Geometry: final body of the model. Coordinates: model frame, mm. Face numbers are marked on the shaded views. A direction names the side the tool comes from. Round coordinates to 2 decimals unless told otherwise and drop trailing zeros. Order: outer loops, then holes, each group sorted by start corner. A loop starts at its lowest first (then second) coordinate and runs counter-clockwise, first axis right, second up. Notation, with made-up numbers: (-8.75, 79) -> (23.25, 79) arc R30 ccw to (23.25, 117) -> close; hole circle Ø8 at (83, 64). An arc over 180 degrees is marked (long way). Put each result on its own line as item: value.
```python
from build123d import *

# Parameters (mm, degrees)
F1_DEPTH = 10
F2_DEPTH = 50
F3_DEPTH = 10
F4_START = 50
F4_DEPTH = 10


# Not quite as in the source:
# - a feature names something its author has since deleted; it is built from what else it names


with BuildPart() as f1:
    # F0 (on Top) → F1 (new body)
    with BuildSketch(Plane.XY):
        with BuildLine():
            Line((0, 11.5), (0, 14))
            ThreePointArc((0, 14), (-14, 0), (0, -14))
            Line((0, -14), (0, -11.5))
            ThreePointArc((0, -11.5), (-2.4269719101, -11.2409878279), (-4.7446194261, -10.4756186692))
            ThreePointArc((-4.7446194261, -10.4756186692), (-8.9623106012, -8.9623106012), (-10.4756186692, -4.7446194261))
            ThreePointArc((-10.4756186692, -4.7446194261), (-11.5, 0), (-10.4756186692, 4.7446194261))
            ThreePointArc((-10.4756186692, 4.7446194261), (-8.9623106012, 8.9623106012), (-4.7446194261, 10.4756186692))
            ThreePointArc((-4.7446194261, 10.4756186692), (-2.4269719101, 11.2409878279), (0, 11.5))
        make_face()
        with BuildLine():
            ThreePointArc((-4.7446194261, -10.4756186692), (-2.4269719101, -11.2409878279), (0, -11.5))
            Line((0, -11.5), (0, -9))
            Line((0, -9), (0, -5.25))
            ThreePointArc((0, -5.25), (-1.3631151282, -8.7791112186), (-4.7446194261, -10.4756186692))
        make_face()
        with BuildLine():
            Line((-5.25, -5.25), (0, -5.25))
            ThreePointArc((0, -5.25), (-0.001489151, -5.124964534), (-0.0059557591, -5))
            Line((-0.0059557591, -5), (-3, -5))
            Line((-3, -5), (-3, -0.5065835097))
            ThreePointArc((-3, -0.5065835097), (-4.0968383837, -0.1282114172), (-5.2499999999, 0))
            Line((-5.25, 0), (-5.25, -5.25))
        make_face()
        with BuildLine():
            ThreePointArc((-10.4756186692, -4.7446194261), (-8.1317279836, -8.1317279836), (-4.7446194261, -10.4756186692))
            ThreePointArc((-4.7446194261, -10.4756186692), (-1.3631151282, -8.7791112186), (0, -5.25))
            Line((0, -5.25), (-5.25, -5.25))
            Line((-5.25, -5.25), (-5.25, 0))
            ThreePointArc((-5.2499999999, 0), (-8.7791112186, -1.3631151282), (-10.4756186692, -4.7446194261))
        make_face()
        with BuildLine():
            ThreePointArc((-5.2499999999, 0), (-8.7791112186, 1.3631151282), (-10.4756186692, 4.7446194261))
            ThreePointArc((-10.4756186692, 4.7446194261), (-11.5, 0), (-10.4756186692, -4.7446194261))
            ThreePointArc((-10.4756186692, -4.7446194261), (-8.7791112186, -1.3631151282), (-5.2499999999, 0))
        make_face()
        with BuildLine():
            ThreePointArc((-3, 0.5065835097), (-4.0968383837, 0.1282114172), (-5.2499999999, 0))
            ThreePointArc((-5.2499999999, 0), (-4.0968383837, -0.1282114172), (-3, -0.5065835097))
            Line((-3, -0.5065835097), (-3, 0.5065835097))
        make_face()
        with BuildLine():
            ThreePointArc((0, 5.25), (-1.3631151282, 8.7791112186), (-4.7446194261, 10.4756186692))
            ThreePointArc((-4.7446194261, 10.4756186692), (-8.1317279836, 8.1317279836), (-10.4756186692, 4.7446194261))
            ThreePointArc((-10.4756186692, 4.7446194261), (-8.7791112186, 1.3631151282), (-5.2499999999, 0))
            Line((-5.25, 0), (-5.25, 5.25))
            Line((-5.25, 5.25), (0, 5.25))
        make_face()
        with BuildLine():
            Line((0, 9), (0, 11.5))
            ThreePointArc((0, 11.5), (-2.4269719101, 11.2409878279), (-4.7446194261, 10.4756186692))
            ThreePointArc((-4.7446194261, 10.4756186692), (-1.3631151282, 8.7791112186), (0, 5.25))
            Line((0, 5.25), (0, 6))
            Line((0, 6), (0, 9))
        make_face()
        with BuildLine():
            ThreePointArc((-10.4756186692, 4.7446194261), (-8.1317279836, 8.1317279836), (-4.7446194261, 10.4756186692))
            ThreePointArc((-4.7446194261, 10.4756186692), (-8.9623106012, 8.9623106012), (-10.4756186692, 4.7446194261))
        make_face()
        with BuildLine():
            ThreePointArc((-10.4756186692, -4.7446194261), (-8.9623106012, -8.9623106012), (-4.7446194261, -10.4756186692))
            ThreePointArc((-4.7446194261, -10.4756186692), (-8.1317279836, -8.1317279836), (-10.4756186692, -4.7446194261))
        make_face()
        with BuildLine():
            ThreePointArc((-0.0059557591, 5), (-0.001489151, 5.124964534), (0, 5.25))
            Line((0, 5.25), (-5.25, 5.25))
            Line((-5.25, 5.25), (-5.25, 0))
            ThreePointArc((-5.2499999999, 0), (-4.0968383837, 0.1282114172), (-3, 0.5065835097))
            Line((-3, 0.5065835097), (-3, 5))
            Line((-3, 5), (-0.0059557591, 5))
        make_face()
    extrude(amount=-F1_DEPTH)

    # F0 (on Top) → F2 (join)
    with BuildSketch(Plane.XY):
        with BuildLine():
            Line((0, 11.5), (0, 14))
            ThreePointArc((0, 14), (-14, 0), (0, -14))
            Line((0, -14), (0, -11.5))
            ThreePointArc((0, -11.5), (-2.4269719101, -11.2409878279), (-4.7446194261, -10.4756186692))
            ThreePointArc((-4.7446194261, -10.4756186692), (-8.9623106012, -8.9623106012), (-10.4756186692, -4.7446194261))
            ThreePointArc((-10.4756186692, -4.7446194261), (-11.5, 0), (-10.4756186692, 4.7446194261))
            ThreePointArc((-10.4756186692, 4.7446194261), (-8.9623106012, 8.9623106012), (-4.7446194261, 10.4756186692))
            ThreePointArc((-4.7446194261, 10.4756186692), (-2.4269719101, 11.2409878279), (0, 11.5))
        make_face()
    extrude(amount=F2_DEPTH)

    # F3 (add): a face of the model
    f3_faces = [f1.faces().sort_by_distance(p)[0] for p in [
        (-2.4930382043, 11.5469865939, 50),
    ]]
    extrude(f3_faces, amount=F3_DEPTH)

    # F0 (on Top) → F4 (join)
    with BuildSketch(Plane.XY.offset(F4_START)):
        with BuildLine():
            Line((0, 9), (0, 11.5))
            ThreePointArc((0, 11.5), (-2.4269719101, 11.2409878279), (-4.7446194261, 10.4756186692))
            ThreePointArc((-4.7446194261, 10.4756186692), (-1.3631151282, 8.7791112186), (0, 5.25))
            Line((0, 5.25), (0, 6))
            Line((0, 6), (0, 9))
        make_face()
        with BuildLine():
            ThreePointArc((-4.7446194261, -10.4756186692), (-2.4269719101, -11.2409878279), (0, -11.5))
            Line((0, -11.5), (0, -9))
            Line((0, -9), (0, -5.25))
            ThreePointArc((0, -5.25), (-1.3631151282, -8.7791112186), (-4.7446194261, -10.4756186692))
        make_face()
        with BuildLine():
            ThreePointArc((0, 5.25), (-1.3631151282, 8.7791112186), (-4.7446194261, 10.4756186692))
            ThreePointArc((-4.7446194261, 10.4756186692), (-8.1317279836, 8.1317279836), (-10.4756186692, 4.7446194261))
            ThreePointArc((-10.4756186692, 4.7446194261), (-8.7791112186, 1.3631151282), (-5.2499999999, 0))
            Line((-5.25, 0), (-5.25, 5.25))
            Line((-5.25, 5.25), (0, 5.25))
        make_face()
        with BuildLine():
            ThreePointArc((-10.4756186692, 4.7446194261), (-8.1317279836, 8.1317279836), (-4.7446194261, 10.4756186692))
            ThreePointArc((-4.7446194261, 10.4756186692), (-8.9623106012, 8.9623106012), (-10.4756186692, 4.7446194261))
        make_face()
        with BuildLine():
            ThreePointArc((-10.4756186692, -4.7446194261), (-8.9623106012, -8.9623106012), (-4.7446194261, -10.4756186692))
            ThreePointArc((-4.7446194261, -10.4756186692), (-8.1317279836, -8.1317279836), (-10.4756186692, -4.7446194261))
        make_face()
        with BuildLine():
            ThreePointArc((-10.4756186692, -4.7446194261), (-8.1317279836, -8.1317279836), (-4.7446194261, -10.4756186692))
            ThreePointArc((-4.7446194261, -10.4756186692), (-1.3631151282, -8.7791112186), (0, -5.25))
            Line((0, -5.25), (-5.25, -5.25))
            Line((-5.25, -5.25), (-5.25, 0))
            ThreePointArc((-5.2499999999, 0), (-8.7791112186, -1.3631151282), (-10.4756186692, -4.7446194261))
        make_face()
        with BuildLine():
            ThreePointArc((-5.2499999999, 0), (-8.7791112186, 1.3631151282), (-10.4756186692, 4.7446194261))
            ThreePointArc((-10.4756186692, 4.7446194261), (-11.5, 0), (-10.4756186692, -4.7446194261))
            ThreePointArc((-10.4756186692, -4.7446194261), (-8.7791112186, -1.3631151282), (-5.2499999999, 0))
        make_face()
        with BuildLine():
            ThreePointArc((-0.0059557591, 5), (-0.001489151, 5.124964534), (0, 5.25))
            Line((0, 5.25), (-5.25, 5.25))
            Line((-5.25, 5.25), (-5.25, 0))
            ThreePointArc((-5.2499999999, 0), (-4.0968383837, 0.1282114172), (-3, 0.5065835097))
            Line((-3, 0.5065835097), (-3, 5))
            Line((-3, 5), (-0.0059557591, 5))
        make_face()
        with BuildLine():
            ThreePointArc((-0.0059557591, -5), (-0.001489151, -5.124964534), (0, -5.25))
            Line((0, -5.25), (0, -5))
            Line((0, -5), (-0.0059557591, -5))
        make_face()
        with BuildLine():
            Line((-5.25, -5.25), (0, -5.25))
            ThreePointArc((0, -5.25), (-0.001489151, -5.124964534), (-0.0059557591, -5))
            Line((-0.0059557591, -5), (-3, -5))
            Line((-3, -5), (-3, -0.5065835097))
            ThreePointArc((-3, -0.5065835097), (-4.0968383837, -0.1282114172), (-5.2499999999, 0))
            Line((-5.25, 0), (-5.25, -5.25))
        make_face()
        with BuildLine():
            ThreePointArc((-3, 0.5065835097), (-4.0968383837, 0.1282114172), (-5.2499999999, 0))
            ThreePointArc((-5.2499999999, 0), (-4.0968383837, -0.1282114172), (-3, -0.5065835097))
            Line((-3, -0.5065835097), (-3, 0.5065835097))
        make_face()
        with BuildLine():
            Line((0, 0), (0, 5))
            Line((0, 5), (-0.0059557591, 5))
            ThreePointArc((-0.0059557591, 5), (-0.8810329928, 2.3388786885), (-3, 0.5065835097))
            Line((-3, 0.5065835097), (-3, -0.5065835097))
            ThreePointArc((-3, -0.5065835097), (-0.8810329928, -2.3388786885), (-0.0059557591, -5))
            Line((-0.0059557591, -5), (0, -5))
            Line((0, -5), (0, 0))
        make_face()
        with BuildLine():
            ThreePointArc((-3, 0.5065835097), (-0.8810329928, 2.3388786885), (-0.0059557591, 5))
            Line((-0.0059557591, 5), (-3, 5))
            Line((-3, 5), (-3, 0.5065835097))
        make_face()
        with BuildLine():
            Line((-3, -5), (-0.0059557591, -5))
            ThreePointArc((-0.0059557591, -5), (-0.8810329928, -2.3388786885), (-3, -0.5065835097))
            Line((-3, -0.5065835097), (-3, -5))
        make_face()
    extrude(amount=F4_DEPTH)


solid = f1.part
```
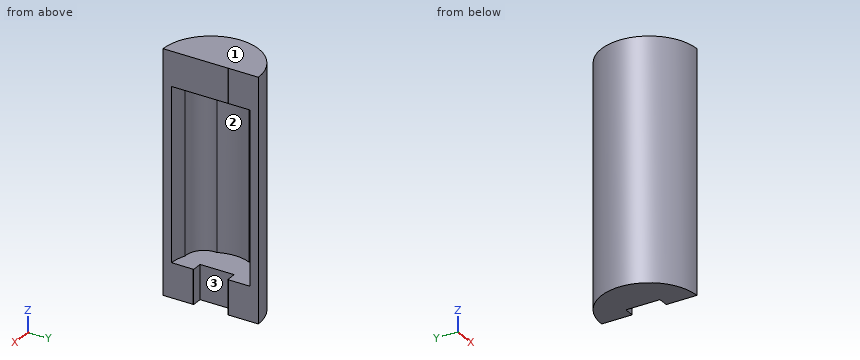
1. Material intervals for probe 1 along Z at (x, y) = (-9.5, 1.5); probe 2 along Y at (x, z) = (-8.5, 39.5); probe 3 along Y at (x, z) = (-3.75, 20.5), sorted ascending.
Ans:
probe 1: -10 to 0, 50 to 60
probe 2: -11.12 to -9.37, 9.37 to 11.12
probe 3: -13.49 to -10.87, 10.87 to 13.49
2. Cut plane D-D on x = -7.75. Return loops of the section in (y, z).
Ans:
outline: (-11.66, -10) -> (11.66, -10) -> (11.66, 60) -> (-11.66, 60) -> close; hole (-9.87, 0) -> (9.87, 0) -> (9.87, 50) -> (-9.87, 50) -> close
3. Cut plane B-B on z = 11.5. Return loops of the section in (x, y), and give its area (3 significant figures).
Ans:
outline: (-10.48, -4.74) arc R11.5 cw to (-10.48, 4.74) arc R5.25 cw to (-4.74, 10.48) arc R11.5 cw to (0, 11.5) -> (0, 14) arc R14 ccw to (0, -14) -> (0, -11.5) arc R11.5 cw to (-4.74, -10.48) arc R5.25 cw to start
area: 86.6 mm²
4. Cut plane A-A on y = 0. Return loops of the section in (x, z).
Ans:
outline: (-14, -10) -> (-3, -10) -> (-3, 0) -> (-11.5, 0) -> (-11.5, 50) -> (0, 50) -> (0, 60) -> (-14, 60) -> close
5. Contact query for flat-ended pins moving along their axis: P1, Ø3, axis at y = 1.5, z = -5, coming from the +X side; P2, Ø8, axis at x = -11.5, z = 44.5, coming from the -Y side; P3, Ø1.5, axis at x = -1, z = -3, coming from the +Y side; P4, Ø2.5, axis at x = -1, z = -4.5, coming from the -Y side. Output: stop coordinate, or through.
Ans:
P1: x = -3
P2: y = -11.82
P3: y = 14
P4: y = -14
6. Set-up query: the marked faces 1, 2 and 3. Return all of +Z, -Z, +X, -X, +Y, -Y with unobstructed straight access to the full face (end or side cutting, diameter ignored); none if empty.
Ans:
face 1: +Z, +X, -X, +Y, -Y
face 2: +X
face 3: -Z, +X
7. Cut plane C-C on x = -3.75. Return loops of the section in (y, z), and give its area (3 significant figures).
Ans:
outline: (-13.49, -10) -> (13.49, -10) -> (13.49, 60) -> (-13.49, 60) -> close; hole (-10.87, 0) -> (10.87, 0) -> (10.87, 50) -> (-10.87, 50) -> close
area: 801 mm²
